For this review, take the finished solid that the model builds, in its own axes (mm). Face numbers are marked on the shaded views. A direction names the side the tool comes from. Give positions to 0.01 mm unless a question says otherwise; leave off trailing zeros. Loops run counter-clockwise (first coordinate to the right, second up) from the corner with the lowest first, then second, coordinate; pieces in that order, holes last.
```python
from build123d import *

# Parameters (mm, degrees)
SKETCH1_R           = 2
BOSS_EXTRUDE1_DEPTH = 5
SKETCH3_R           = 2
BOSS_EXTRUDE2_DEPTH = 10
SKETCH4_W           = 24.111622735
SKETCH4_H           = 4.195341451
CUT_EXTRUDE1_DEPTH  = 16


with BuildPart() as part:
    # Sketch1 → Boss-Extrude1 (new body)
    with BuildSketch(Plane(origin=(0, 0, 0), x_dir=(1, 0, 0), z_dir=(0, 1, 0))):
        with BuildLine():
            Line((0, 0), (30, 0))
            ThreePointArc((30, 0), (37.5, 7.5), (30, 15))
            Line((30, 15), (0, 15))
            ThreePointArc((0, 15), (-7.5, 7.5), (0, 0))
        make_face()
        with Locations((0, 7.5)):
            Circle(SKETCH1_R, mode=Mode.SUBTRACT)
        with Locations((30, 7.5)):
            Circle(SKETCH1_R, mode=Mode.SUBTRACT)
    extrude(amount=BOSS_EXTRUDE1_DEPTH)

    # Sketch3 → Boss-Extrude2 (add)
    with BuildSketch(Plane(origin=(0, 0, -15), x_dir=(-1, 0, 0), z_dir=(0, 0, -1))):
        with BuildLine():
            Line((-22.5, 5), (-7.5, 5))
            Line((-7.5, 5), (-7.5, 21.75))
            ThreePointArc((-7.5, 21.75), (-15, 29.25), (-22.5, 21.75))
            Line((-22.5, 21.75), (-22.5, 5))
        make_face()
        with Locations((-15, 21.75)):
            Circle(SKETCH3_R, mode=Mode.SUBTRACT)
    extrude(amount=-BOSS_EXTRUDE2_DEPTH)

    # Sketch4 → Cut-Extrude1 (cut, through all)
    with BuildSketch(Plane(origin=(0, 0, -15), x_dir=(-1, 0, 0), z_dir=(0, 0, -1))):
        with Locations((-13.441214338, 29.097670726)):
            Rectangle(SKETCH4_W, SKETCH4_H)
    extrude(amount=-CUT_EXTRUDE1_DEPTH, mode=Mode.SUBTRACT)


solid = part.part
```
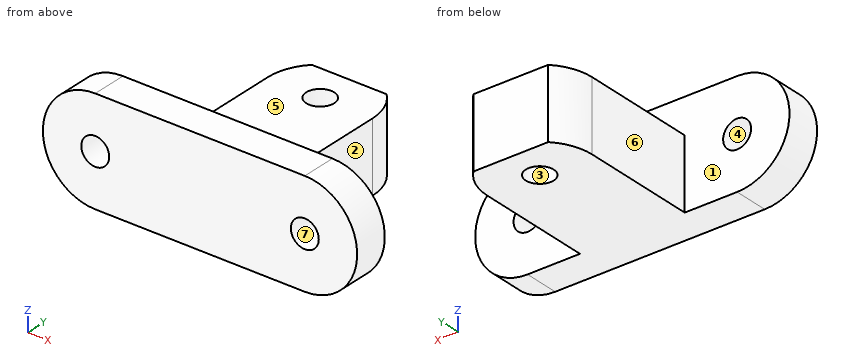
Item 1: Take a section at A-A on z = -7.5. Give the boundary of the cut face in (x, y), and give its area (3 significant figures).
Answer:
outline: (-7.5, 0) - (-2, 0) - (-2, 5) - (-7.5, 5) - close; (2, 0) - (28, 0) - (28, 5) - (22.5, 5) - (22.5, 21.75) arc R7.5 ccw to (20.36, 27) - (9.64, 27) arc R7.5 ccw to (7.5, 21.75) - (7.5, 5) - (2, 5) - close; (32, 0) - (37.5, 0) - (37.5, 5) - (32, 5) - close; hole circle Ø4 at (15, 21.75)
area: 495 mm2
Item 2: Take a section at D-D on x = -0.5. Give the boundary of the cut face in (y, z).
Answer:
outline: (0, -14.98) - (5, -14.98) - (5, -9.44) - (0, -9.44) - close; (0, -5.56) - (5, -5.56) - (5, -0.02) - (0, -0.02) - close
Item 3: Take a section at B-B on x = 15. Give the boundary of the cut face in (y, z).
Answer:
outline: (0, -15) - (19.75, -15) - (19.75, -5) - (5, -5) - (5, 0) - (0, 0) - close; (23.75, -15) - (27, -15) - (27, -5) - (23.75, -5) - close
Item 4: Clearance check with flat-ended pins moving along their axes: pin 1 Ø8 at (y, z) = (10.5, -11) entering from +X; pin 2 Ø3 at (x, y) = (15, 21.75) entering from +Z; pin 3 Ø5 at (x, z) = (0, -7.5) entering from +Y; pin 4 Ø8 at (y, z) = (14, -12) entering from -X. State where each tip first meets the part, or that it passes through.
Answer:
pin 1: stops at x = 22.5
pin 2: passes through
pin 3: stops at y = 5
pin 4: stops at x = 7.5
Item 5: For L1, parallel to X at y = 2, z = -7.5; L2, parallel to Y at x = 15, z = -13.75; L3, parallel to Z at x = 30, y = 3.7, list the stretches that pass through material, from the lowest coordinate up.
Answer:
L1: x = -7.5 to -2, 2 to 28, 32 to 37.5
L2: y = 0 to 19.75, 23.75 to 27
L3: z = -15 to -9.5, -5.5 to 0
Item 6: Take a section at C-C on y = 21.25. Give the boundary of the cut face in (x, z), and give its area (3 significant figures).
Answer:
outline: (7.5, -15) - (13.06, -15) - (13.06, -5) - (7.5, -5) - close; (16.94, -15) - (22.5, -15) - (22.5, -5) - (16.94, -5) - close
area: 111 mm2
Item 7: The part is to be moulded in two halves that separate along X. For the marked faces 1, 2, 3 and 4, say which applies: released by +X, released by -X, zero draft, split by the parting line, or undercut.
Answer:
face 1: zero draft
face 2: released by +X
face 3: undercut
face 4: undercut
Item 8: Tool access review of the marked faces 5, 6 and 7: name each direction out of +Z, -Z, +X, -X, +Y, -Y from which nothing blocks a thin tool from reaching the whole face with its end or side.
Answer:
face 5: +Z, +X, -X, +Y
face 6: +Z, -Z, -X, +Y
face 7: +Y, -Y
